Could you check a few things on this model? Use its own coordinates, in mm. Face numbers are marked on the shaded views. A direction names the side the tool comes from. Round coordinates to 2 decimals unless told otherwise and drop trailing zeros. Write each loop counter-clockwise with the first axis right and the second up, starting at its lowest first coordinate (ties: lowest second). Pieces come first, ordered by that corner, then holes. Notation, with made-up numbers: (85.25, 40) -> (125.25, 40) arc R23 cw to (125.25, 59) -> close; hole circle Ø1 at (66, 39.5). An arc over 180 degrees is marked (long way). Answer in a Markdown table with one row per item.
from build123d import *

# Parameters (mm, degrees)
F4_R = 6


with BuildPart() as f1:
    # F0 (on Front) → F1 (revolve)
    with BuildSketch(Plane.XZ):
        with BuildLine():
            Line((0, 62), (0, 0))
            Line((0, 0), (88, 0))
            Line((88, 0), (88, 32))
            Line((88, 32), (85, 32))
            Line((85, 32), (85, 40))
            Line((85, 40), (68, 40))
            Line((68, 40), (68, 62))
            Line((68, 62), (54.569368, 62))
            ThreePointArc((54.569368, 62), (48.569368, 56), (42.569368, 62))
            Line((42.569368, 62), (0, 62))
        make_face()
    revolve(axis=Axis((-15.071996, 0, 0), (-1, 0, 0)))

    # F2 (on Front) → F3 (revolve, cut)
    with BuildSketch(Plane.XZ):
        Polygon((0, 50), (0, 0), (88, 0), (88, 12), (31.5, 12), (31.5, 32), (23.5, 32), (23.5, 41), (16.5, 41), (16.5, 22.69382), (13.5, 22.69382), (13.5, 32), (1.5, 32), (1.5, 50), align=None)
    revolve(axis=Axis((-15.359187, 0, 0), (-1, 0, 0)), mode=Mode.SUBTRACT)

    # F4
    f4_edges = [f1.edges().sort_by_distance(p)[0] for p in [
        (0, 0, -62),
    ]]
    fillet(f4_edges, radius=F4_R)


solid = f1.part
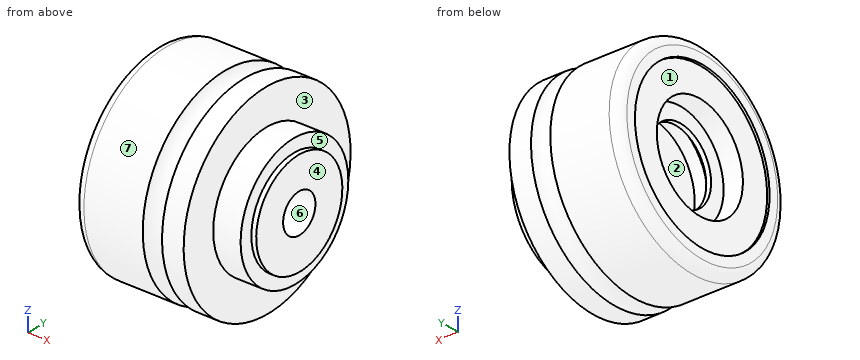
1) For the marked faces 1, 2, 3 and 4, which set-ups out of +Z, -Z, +X, -X, +Y, -Y let a thin tool reach every point of the face, with its end or its side?
Findings:
| item | result |
|---|---|
| face 1 | -X |
| face 2 | none |
| face 3 | +X |
| face 4 | +Z, -Z, +X, +Y, -Y |
2) Thinking about a two-plate mould opening in Z: for the marked faces 5, 6 and 7, which applies, +Z half, -Z half, draft (parallel to the pull), parting line (faces both ways), or undercut?
Findings:
| item | result |
|---|---|
| face 5 | draft |
| face 6 | undercut |
| face 7 | parting line |
3) Imagine slicing it at A-A, the plane x = 35. Please give me the cut outline in (y, z), plus the area to 3 significant figures.
Findings:
| item | result |
|---|---|
| outline | circle Ø124 at (0, 0); hole circle Ø24 at (0, 0) |
| area | 11,600 mm^2 |
4) Imagine slicing it at B-B, the plane x = 46.5. Please give me the cut outline in (y, z), plus the area to 3 significant figures.
Findings:
| item | result |
|---|---|
| outline | circle Ø112.74 at (0, 0); hole circle Ø24 at (0, 0) |
| area | 9,530 mm^2 |
5) Please list where these lines run through material, in increasing order: line 1 (Y direction, x = 15, z = 0); line 2 (Y direction, x = 30, z = 0); line 3 (X direction, y = 14, z = 21.5).
Findings:
| item | result |
|---|---|
| line 1 | y = -62 to -22.69, 22.69 to 62 |
| line 2 | y = -62 to -32, 32 to 62 |
| line 3 | x = 13.5 to 16.5, 31.5 to 88 |
6) For pin 1 (10 mm diameter, centred on x = 78.5, z = -18, fed in from +Y); pin 2 (5 mm diameter, centred on x = 66, z = -4, fed in from -Y); pin 3 (1 mm diameter, centred on x = 38, z = -39, fed in from +Y); pin 4 (6 mm diameter, centred on y = -1.5, z = 49.5, fed in from -X), each with a flat end and sliding along its axis, tell me the tip position at first contact or that it passes through.
Findings:
| item | result |
|---|---|
| pin 1 | stops at y = 37.83 |
| pin 2 | stops at y = -61.98 |
| pin 3 | stops at y = 48.6 |
| pin 4 | stops at x = 0 |
